from build123d import *

# Parameters (mm, degrees)
F0_W          = 25
F0_H          = 80
F0_R          = 4.25
F1_DEPTH      = 20
F1_DEPTH_BACK = 20
F2_R          = 4.25
F3_DEPTH      = 12.5
F4_R          = 11
F5_DEPTH      = 10
F6_R          = 4.25
F7_DEPTH      = 25


with BuildPart() as f1:
    # F0 (on Front) → F1 (new body, two sides)
    with BuildSketch(Plane.XZ) as f1_sk:
        Rectangle(F0_W, F0_H)
        with Locations((0, -27.5)):
            Circle(F0_R, mode=Mode.SUBTRACT)
        with Locations((0, 27.5)):
            Circle(F0_R, mode=Mode.SUBTRACT)
    extrude(amount=F1_DEPTH)
    extrude(f1_sk.sketch, amount=-F1_DEPTH_BACK)

    # F2 (on Right) → F3 (cut, through all)
    with BuildSketch(Plane.YZ):
        Circle(F2_R)
    extrude(amount=-F3_DEPTH, mode=Mode.SUBTRACT)

    # F4 (on face) → F5 (cut)
    with BuildSketch(Plane.YZ.offset(12.5)):
        Circle(F4_R)
    extrude(amount=-F5_DEPTH, mode=Mode.SUBTRACT)

    # F6 (on face) → F7 (cut)
    with BuildSketch(Plane.YZ.offset(12.5)):
        Circle(F6_R)
    extrude(amount=-F7_DEPTH, mode=Mode.SUBTRACT)


solid = f1.part
Geometry check sheet. Reference: the model listing, model coordinates, mm. A direction names the side the tool comes from. Give positions to 0.01 mm unless a question says otherwise; leave off trailing zeros. Loops run counter-clockwise (first coordinate to the right, second up) from the corner with the lowest first, then second, coordinate; pieces in that order, holes last. Notation, with made-up numbers: (42, 87) -> (98, 87) arc R20 ccw to (98, 97) -> close; hole circle Ø7 at (55, -22). An arc over 180 degrees is marked (long way). Answer in a Markdown table with one row per item. Add a question column.
1) Draft check along X on faces 1 (the face through (-12.5, -5, -1)), 2 (the face through (2.285, 0.28, 31.084)), 3 (the face through (0, 0, -40)), 4 (the face through (2.5, 0, -5)). Enter one of: pulls with the +X half, pulls with the -X half, needs draft (parallel to the pull), parting line crosses it, or undercut.
2) Cross-section at B-B on x = 0. Record the boundary of the cut face in (y, z), and give its area (3 significant figures).
3) Cross-section at D-D on y = -16. Record the boundary of the cut face in (x, z).
4) Material ranges on probe 1 along Z at (x, y) = (0.25, 16); probe 2 along Z at (x, y) = (1.75, 13.5); probe 3 along X at (y, z) = (1, 10.5), recorded low to high. Write a range as from..to.
5) Gauge pin test, flat ends, axial feed: P1, Ø13.5, axis at y = 0, z = 0, coming from the +X side; P2, Ø5, axis at x = 0, z = 27.5, coming from the +Y side; P3, Ø13.5, axis at x = 0, z = -27.5, coming from the -Y side. Record the tip position at first contact, or that the pin passes through.
6) Cross-section at A-A on y = 0. Record the boundary of the cut face in (x, z), and give its area (3 significant figures).
7) Set-up check for faces 5 (the face through (-4.895, 2.285, 3.584)), 6 (the face through (7.57, -2.38, -10.74)): record each of +Z, -Z, +X, -X, +Y, -Y from which the full face is reachable in a straight line by a thin tool's end or side.
8) Cross-section at C-C on z = -27.5. Record the boundary of the cut face in (x, y), and give its area (3 significant figures).
Outcome:
| question | item | result |
|---|---|---|
| 1 | face 1 | pulls with the -X half |
| 1 | face 2 | undercut |
| 1 | face 3 | needs draft |
| 1 | face 4 | pulls with the +X half |
| 2 | outline | (-20, -40) -> (20, -40) -> (20, -31.75) -> (-20, -31.75) -> close; (-20, -23.25) -> (20, -23.25) -> (20, 23.25) -> (-20, 23.25) -> close; (-20, 31.75) -> (20, 31.75) -> (20, 40) -> (-20, 40) -> close; hole circle Ø8.5 at (0, 0) |
| 2 | area | 2,460 mm^2 |
| 3 | outline | (-12.5, -40) -> (12.5, -40) -> (12.5, 40) -> (-12.5, 40) -> close; hole circle Ø8.5 at (0, -27.5); hole circle Ø8.5 at (0, 27.5) |
| 4 | probe 1 | z = -40..-31.74, -23.26..23.26, 31.74..40 |
| 4 | probe 2 | z = -40..-31.37, -23.63..23.63, 31.37..40 |
| 4 | probe 3 | x = -12.5..2.5 |
| 5 | P1 | stops at x = 2.5 |
| 5 | P2 | passes through |
| 5 | P3 | stops at y = -20 |
| 6 | outline | (-12.5, -40) -> (12.5, -40) -> (12.5, -11) -> (2.5, -11) -> (2.5, -4.25) -> (-12.5, -4.25) -> close; (-12.5, 4.25) -> (2.5, 4.25) -> (2.5, 11) -> (12.5, 11) -> (12.5, 40) -> (-12.5, 40) -> close; hole circle Ø8.5 at (0, -27.5); hole circle Ø8.5 at (0, 27.5) |
| 6 | area | 1,540 mm^2 |
| 7 | face 5 | +X, -X |
| 7 | face 6 | +X |
| 8 | outline | (-12.5, -20) -> (-4.25, -20) -> (-4.25, 20) -> (-12.5, 20) -> close; (4.25, -20) -> (12.5, -20) -> (12.5, 20) -> (4.25, 20) -> close |
| 8 | area | 660 mm^2 |
